Autodesk Inventor part; units mm, degrees
sketch "スケッチ1" plane through (0, 0, 0) normal (0, 0, 1) x (1, 0, 0)
  line L0 (-5.1, 4.8) -> (5.1, 4.8)
  line L1 (5.1, 4.8) -> (5.1, -4.8)
  line L2 (5.1, -4.8) -> (-5.1, -4.8)
  line L3 (-5.1, -4.8) -> (-5.1, 4.8)
  point P0 (0, 0)
  dimension "d0" = 4.8
  dimension "d1" = 4.8
  dimension "d2" = 5.1
  dimension "d3" = 5.1
extrude "押し出し1" add sketch "スケッチ1" along normal blind 1.6 and the other way blind 3.6
sketch "スケッチ2" plane through (0, 0, -3.6) normal (0, 0, -1) x (-1, 0, 0)
  line L0 (5.1, 4.8) -> (-5.1, 4.8)
  line L1 (-5.1, 4.8) -> (-5.1, -4.8)
  line L2 (-5.1, -4.8) -> (5.1, -4.8)
  line L3 (5.1, -4.8) -> (5.1, 4.8)
  line L4 (5.1, -6.8) -> (-5.1, -6.8)
  line L5 (-5.1, -6.8) -> (-5.1, 6.8)
  line L6 (-5.1, 6.8) -> (5.1, 6.8)
  line L7 (5.1, 6.8) -> (5.1, -6.8)
  line L8 (0, -9.52) -> (0, 9.52)
  point P0 (0, 0)
  dimension "d8" = 2
  dimension "d24" = 5.1
  dimension "d30" = 5.1
extrude "押し出し2" add sketch "スケッチ2" against normal blind 1.2 contours L0 L8 L6 L7 | L0 L5 L6 L8 | L7 L4 L8 L2 | L8 L4 L5 L2
sketch "スケッチ3" plane through (0, 0, 0) normal (0, 0, 1) x (1, 0, 0)
  line L0 (5.1, 4.8) -> (-5.1, 4.8)
  line L1 (-5.1, 4.8) -> (-5.1, -4.8)
  line L2 (-5.1, -4.8) -> (5.1, -4.8)
  line L3 (5.1, -4.8) -> (5.1, 4.8)
  circle A0 centre (0, 0) radius 3.25
  dimension "d28" = 6.5
extrude "押し出し3" cut sketch "スケッチ3" against normal through all contours A0
fillet "フィレット2" radius 2 4 edges at (5.1, -4.8, -0.4) (5.1, 4.8, -0.4) (-5.1, 4.8, -0.4) (-5.1, -4.8, -0.4)
fillet "フィレット3" radius 1 4 edges at (5.1, -6.8, -3) (-5.1, -6.8, -3) (5.1, 6.8, -3) (-5.1, 6.8, -3)
properties part number "HbBatteryLockKnob01"
Check sheet for the modelled part. Datum: model origin and axes. Units: mm. A direction names the side the tool comes from. Round coordinates to 2 decimals unless told otherwise and drop trailing zeros. Loops run counter-clockwise (first coordinate to the right, second up) from the corner with the lowest first, then second, coordinate; pieces in that order, holes last. Notation, with made-up numbers: (-28.5, -26) - (-20.5, -26) arc R18 ccw to (-20.5, -21) - close; hole circle Ø6 at (-35, -30). An arc over 180 degrees is marked (long way). Answer as CSV lines item,"result". Start each with the question number.
Item 1: Scan lines: line 1 (Y direction, x = 0, z = -1.5); line 2 (Y direction, x = 0, z = -2.6); line 3 (Z direction, x = 0, y = -3). Record each from-to range of solid material in increasing order. Write a range as [from, to].
Item 2: Release check for a two-part mould opening along Y. For faces 5 (the cylindrical face through (4.5, 4.23, -0.43)), 6 (the cylindrical face through (-2.579, -1.978, -1.775)), 7 (the cylindrical face through (4.799, -6.515, -2.992)) record: +Y half, -Y half, draft (parallel to the pull), parting line (faces both ways), or undercut.
Item 3: Section check D-D (z = 1). Record the boundary of the cut face in (x, y).
Item 4: Section check A-A (z = -1). Record the boundary of the cut face in (x, y), and give its area (3 significant figures).
Item 5: Section check B-B (x = 0). Record the boundary of the cut face in (y, z).
Item 6: Set-up check for faces 1 (the cylindrical face through (-4.5, 4.23, -0.37)), 2 (the flat face through (0, 4.8, 0)), 3 (the flat face through (0, 0, 0)), 4 (the flat face through (0, -4.8, 0)): record each of +Z, -Z, +X, -X, +Y, -Y from which the full face is reachable in a straight line by a thin tool's end or side.
Item 7: Section check C-C (y = 0). Record the boundary of the cut face in (x, z), and give its area (3 significant figures).
Item 8: Depth check by flat-ended pin: P1, Ø2, axis at x = -2.5, z = -2, coming from the -Y side; P2, Ø3, axis at x = -1, z = 0, coming from the -Y side; P3, Ø1.2, axis at x = 0, z = -1, coming from the +Y side. Enter the tip coordinate at first touch or a pass-through.
Report:
1,line 1,"y = [-4.8, -3.25], [3.25, 4.8]"
1,line 2,"y = [-6.8, -3.25], [3.25, 6.8]"
1,line 3,"z = [0, 1.6]"
2,face 5,"+Y half"
2,face 6,"undercut"
2,face 7,"-Y half"
3,outline,"(-5.1, -2.8) arc R2 ccw to (-3.1, -4.8) - (3.1, -4.8) arc R2 ccw to (5.1, -2.8) - (5.1, 2.8) arc R2 ccw to (3.1, 4.8) - (-3.1, 4.8) arc R2 ccw to (-5.1, 2.8) - close"
4,outline,"(-5.1, -2.8) arc R2 ccw to (-3.1, -4.8) - (3.1, -4.8) arc R2 ccw to (5.1, -2.8) - (5.1, 2.8) arc R2 ccw to (3.1, 4.8) - (-3.1, 4.8) arc R2 ccw to (-5.1, 2.8) - close; hole circle Ø6.5 at (0, 0)"
4,area,"61.3 mm2"
5,outline,"(-6.8, -3.6) - (-3.25, -3.6) - (-3.25, 0) - (3.25, 0) - (3.25, -3.6) - (6.8, -3.6) - (6.8, -2.4) - (4.8, -2.4) - (4.8, 1.6) - (-4.8, 1.6) - (-4.8, -2.4) - (-6.8, -2.4) - close"
6,face 1,"+Z, -X, +Y"
6,face 2,"+Z, +X, -X, +Y"
6,face 3,"-Z"
6,face 4,"+Z, +X, -X, -Y"
7,outline,"(-5.1, -3.6) - (-3.25, -3.6) - (-3.25, 0) - (3.25, 0) - (3.25, -3.6) - (5.1, -3.6) - (5.1, 1.6) - (-5.1, 1.6) - close"
7,area,"29.6 mm2"
8,P1,"stops at y = -6.8"
8,P2,"stops at y = -4.8"
8,P3,"stops at y = 4.8"
